Autodesk Inventor part; units mm, degrees
ref_plane "YZ Plane" through (0, 0, 0) normal (1, 0, 0) x (0, 1, 0)
ref_plane "XZ Plane" through (0, 0, 0) normal (0, 1, 0) x (-1, 0, 0)
ref_plane "XY Plane" through (0, 0, 0) normal (0, 0, 1) x (1, 0, 0)
sketch "スケッチ1" plane through (0, 0, 0) normal (0, 0, 1) x (1, 0, 0)
  circle A0 centre (0, 0) radius 17.5 construction
  circle A1 centre (-7, 0) radius 10.5 construction
  circle A2 centre (-7, 0) radius 6
  circle A3 centre (0, 0) radius 6
  line L0 (-7, 6) -> (0, 6)
  line L1 (0, 6) -> (0, -6) construction
  line L2 (0, -6) -> (-7, -6)
  line L3 (-7, -6) -> (-7, 6) construction
  dimension "d2" = 12
  dimension "d3" = 12
  dimension "d0" = 35
  dimension "d1" = 21
extrude "押し出し1" add sketch "スケッチ1" along normal blind 2
sketch "スケッチ2" plane through (0, 0, 2) normal (0, 0, 1) x (1, 0, 0)
  circle A0 centre (0, 0) radius 3
  dimension "d6" = 6
extrude "押し出し2" add sketch "スケッチ2" along normal blind 3
sketch "スケッチ3" plane through (0, 0, 0) normal (0, 0, -1) x (-1, 0, 0)
  arc A0 (7, -6) -> (7, 6) centre (7, 0) ccw
  circle A1 centre (7, 0) radius 3
  point P0 (0, 0)
  dimension "d9" = 6
extrude "押し出し3" add sketch "スケッチ3" along normal blind 3
properties part number "wrist_gear_spacer"
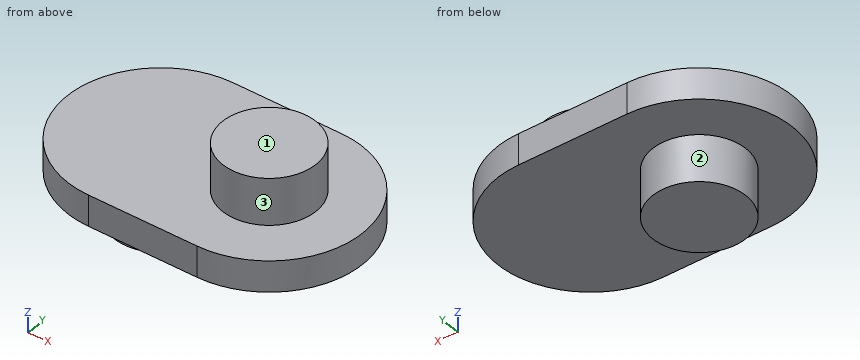
CAD build for the part. Positions are in the model's coordinates, mm. Face numbers are marked on the shaded views. A direction names the side the tool comes from. Give positions to 0.01 mm unless a question says otherwise; leave off trailing zeros. Loops run counter-clockwise (first coordinate to the right, second up) from the corner with the lowest first, then second, coordinate; pieces in that order, holes last. Notation, with made-up numbers: (43, 51.25) -> (80, 51.25) arc R12 cw to (80, 65.25) -> close; hole circle Ø2 at (62.25, 31). An arc over 180 degrees is marked (long way). Use a Markdown table: item, result.
1. Slice it at A-A (x = 2.25). List the corners of the cut face in (y, z).
Check result:
| item | result |
|---|---|
| outline | (-5.56, 0) -> (5.56, 0) -> (5.56, 2) -> (1.98, 2) -> (1.98, 5) -> (-1.98, 5) -> (-1.98, 2) -> (-5.56, 2) -> close |
2. Slice it at C-C (z = 0.5). List the corners of the cut face in (x, y), plus the area to 3 significant figures.
Check result:
| item | result |
|---|---|
| outline | (-7, -6) -> (0, -6) arc R6 ccw to (0, 6) -> (-7, 6) arc R6 ccw to start |
| area | 197 mm^2 |
3. Slice it at D-D (x = -8). List the corners of the cut face in (y, z), plus the area to 3 significant figures.
Check result:
| item | result |
|---|---|
| outline | (-5.92, 0) -> (-2.83, 0) -> (-2.83, -3) -> (2.83, -3) -> (2.83, 0) -> (5.92, 0) -> (5.92, 2) -> (-5.92, 2) -> close |
| area | 40.6 mm^2 |
4. Wall check: L1, parallel to Z at x = -5.75, y = -2; L2, parallel to Z at x = -10.25, y = 4.75; L3, parallel to X at y = -0.25, z = 0.25. Give the ranges that are in metal, low to high. Write a range as [from, to].
Check result:
| item | result |
|---|---|
| L1 | z = [-3, 2] |
| L2 | z = [0, 2] |
| L3 | x = [-12.99, 5.99] |
5. Flat gauge pins, fed straight in: pin 1 (4 mm diameter, centred on x = -5, y = 4.5, fed in from +Z); pin 2 (1 mm diameter, centred on y = 0, z = -1, fed in from +X); pin 3 (1.5 mm diameter, centred on y = 1.5, z = -1.5, fed in from -X). Where does each tip first touch, or does it go through?
Check result:
| item | result |
|---|---|
| pin 1 | stops at z = 2 |
| pin 2 | stops at x = -4 |
| pin 3 | stops at x = -9.9 |
6. Slice it at B-B (y = 2). List the corners of the cut face in (x, z), plus the area to 3 significant figures.
Check result:
| item | result |
|---|---|
| outline | (-12.66, 0) -> (-9.24, 0) -> (-9.24, -3) -> (-4.76, -3) -> (-4.76, 0) -> (5.66, 0) -> (5.66, 2) -> (2.24, 2) -> (2.24, 5) -> (-2.24, 5) -> (-2.24, 2) -> (-12.66, 2) -> close |
| area | 63.5 mm^2 |
7. Which spindle directions (+Z, -Z, +X, -X, +Y, -Y) get a long thin tool onto all of the face, cutting with end or side? Do the marked faces 1, 2 and 3. Say none if no direction does.
Check result:
| item | result |
|---|---|
| face 1 | +Z, +X, -X, +Y, -Y |
| face 2 | -Z |
| face 3 | +Z |
